Check sheet for the modelled part. Datum: model origin and axes. Units: mm. Give positions to 0.01 mm unless a question says otherwise; leave off trailing zeros. One line per item, written item: value. Start each with the question number.
Autodesk Inventor part; units mm, degrees
ref_plane "YZ Plane" through (0, 0, 0) normal (1, 0, 0) x (0, 1, 0)
ref_plane "XZ Plane" through (0, 0, 0) normal (0, 1, 0) x (-1, 0, 0)
ref_plane "XY Plane" through (0, 0, 0) normal (0, 0, 1) x (1, 0, 0)
sketch "Sketch1" plane through (0, 0, 0) normal (0, 1, 0) x (-1, 0, 0)
  line L0 (-105, -105) -> (105, -105)
  line L1 (105, -105) -> (105, 105)
  line L2 (105, 105) -> (-105, 105)
  line L3 (-105, 105) -> (-105, -105)
  line L4 (-105, -105) -> (105, 105) construction
  line L5 (105, -105) -> (-105, 105) construction
  point P0 (0, 0)
  dimension "d0" = 210
extrude "Extrusion1" add sketch "Sketch1" along normal blind 3
sketch "Sketch2" plane through (0, 3, 0) normal (0, 1, 0) x (1, 0, 0)
  line L0 (45.25, 95) -> (-45.25, 95) construction
  line L1 (-45.25, 95) -> (-45.25, -95) construction
  line L2 (-45.25, -95) -> (45.25, -95) construction
  line L3 (45.25, -95) -> (45.25, 95) construction
  line L4 (45.25, 95) -> (-45.25, -95) construction
  line L5 (-45.25, 95) -> (45.25, -95) construction
  point P0 (0, 0)
  dimension "d3" = 190
  dimension "d4" = 90.5
hole "Hole1" at (45.25, 3, 95) at (45.25, 3, -95) at (-45.25, 3, -95) at (-45.25, 3, 95) direction (0, -1, 0) diameter 3.5 end through all countersink diameter 7 countersink angle 90
fillet "Fillet1" radius 3 4 edges at (-105, 1.5, 105) (105, 1.5, 105) (105, 1.5, -105) (-105, 1.5, -105)
properties part number "Stock Build Plate"
1) Draft check along X on faces 1 (the flat face through (1, 3, 1)), 2 (the conical face through (-43.68, 1.36, 96)). Enter one of: released by +X, released by -X, zero draft, split by the parting line, or undercut.
2) Material ranges on L1, parallel to X at y = 0.95, z = 95; L2, parallel to Z at x = 45.25, y = 0.3, recorded low to high. Write a range as from..to.
3) Gauge pin test, flat ends, axial feed: pin 1 (4.5 mm diameter, centred on x = -45.25, z = 95, fed in from +Y); pin 2 (3 mm diameter, centred on x = 45.25, z = 95, fed in from +Y); pin 3 (5.5 mm diameter, centred on x = -45.25, z = -95, fed in from +Y). Record the tip position at first contact, or that the pin passes through.
Data:
1. face 1: zero draft
1. face 2: undercut
2. L1: x = -105..-47, -43.5..43.5, 47..105
2. L2: z = -105..-96.75, -93.25..93.25, 96.75..105
3. pin 1: stops at y = 1.75
3. pin 2: passes through
3. pin 3: stops at y = 2.25
